Can you work these out from the model? Positions are in its coordinate system, mm. A direction names the side the tool comes from. Coordinates: 2 decimals unless noted, no trailing zeros. Order: outer loops, then holes, each group sorted by start corner. A loop starts at its lowest first (then second) coordinate and runs counter-clockwise, first axis right, second up. Notation, with made-up numbers: (29.25, -21.5) -> (83.25, -21.5) arc R24 cw to (83.25, -2.5) -> close; hole circle Ø1 at (63.5, -13.5). An arc over 180 degrees is marked (long way). Use a Markdown table: item, result. Add a question column.
1. Suppose I cut it at A-A, the plane z = 4. List the corners of the cut face in (x, y) for me.
2. We'd pull the mould along X, two halves only. Please class faces 1 (the flat face through (-0.4, 19, 44.4)), 2 (the flat face through (2, 13, 19.05)), 3 (the flat face through (-51.863, 13, 31)): pulls with the +X half, pulls with the -X half, needs draft (parallel to the pull), parting line crosses it, or undercut.
3. For pin 1 Ø1 at (y, z) = (-6, 31) entering from +X; pin 2 Ø21 at (y, z) = (30, 12.5) entering from +X; pin 3 Ø7.5 at (x, y) = (61, 32) entering from +Z; pin 4 Ø12 at (x, z) = (-9.5, 12.5) entering from -Y (1 decimal), each with a flat end and sliding along its axis, tell me the tip position at first contact or that it passes through.
4. Suppose I cut it at B-B, the plane x = 58. List the corners of the cut face in (y, z) for me, then the cut area to 3 significant figures.
5. For faces 4 (the flat face through (59, 41, 12.7)), 5 (the flat face through (62.62, -12.88, 6.26)), 6 (the flat face through (-34.61, 13, 9)), which set-ups out of +Z, -Z, +X, -X, +Y, -Y let a thin tool reach every point of the face, with its end or its side?
6. Suppose I cut it at D-D, the plane x = -38.5. List the corners of the cut face in (y, z) for me.
7. Suppose I cut it at C-C, the plane y = 1.5. List the corners of the cut face in (x, z) for me, then the cut area to 3 significant figures.
8. If I drill on line 1 along X through (y, z) = (2, 14.5); line 2 along X through (y, z) = (-21.5, 35); line 3 along Z through (x, y) = (-59, -8), over which ranges is the centre line in solid material (lowest first)? Write a range as from..to.
```python
from build123d import *

# Parameters (mm, degrees)
F0_W     = 20.847595
F0_H     = 76.2
F1_DEPTH = 12.7
F2_DEPTH = 50.8
F3_DEPTH = 12.7
F4_DEPTH = 12.7
F6_DEPTH = 122.448595
F7_W     = 71.647595
F7_H     = 19.05
F8_DEPTH = 101.6


with BuildPart() as f1:
    # F0 (on Top) → F1 (new body)
    with BuildSketch(Plane.XY):
        with Locations((-62.286463, 12.7)):
            Rectangle(F0_W, F0_H)
    extrude(amount=F1_DEPTH)

    # F0 (on Top) → F2 (join)
    with BuildSketch(Plane.XY):
        Polygon((49.737334, 50.8), (-51.862666, 50.8), (-51.862666, -25.4), (49.737334, -25.4), (49.737334, 0), (49.737334, 25.4), align=None)
    extrude(amount=F2_DEPTH)

    # F0 (on Top) → F3 (join)
    with BuildSketch(Plane.XY):
        Polygon((75.137334, 50.8), (49.737334, 50.8), (49.737334, 25.4), align=None)
    extrude(amount=F3_DEPTH)

    # F0 (on Top) → F4 (join)
    with BuildSketch(Plane.XY):
        Polygon((49.737334, 0), (49.737334, -25.4), (75.137334, -25.4), align=None)
    extrude(amount=F4_DEPTH)

    # F5 (on face) → F6 (cut, through all)
    with BuildSketch(Plane.YZ.offset(49.737334)):
        Polygon((25.4, 50.8), (0, 50.8), (12.7, 38.1), align=None)
    extrude(amount=-F6_DEPTH, mode=Mode.SUBTRACT)

    # F7 (on face) → F8 (cut)
    with BuildSketch(Plane(origin=(0, 50.8, 0), x_dir=(-1, 0, 0), z_dir=(0, 1, 0))):
        with Locations((-1.213537, 9.525)):
            Rectangle(F7_W, F7_H)
    extrude(amount=-F8_DEPTH, mode=Mode.SUBTRACT)


solid = f1.part
```
Worked out:
| question | item | result |
|---|---|---|
| 1 | outline | (-72.71, -25.4) -> (-34.61, -25.4) -> (-34.61, 50.8) -> (-72.71, 50.8) -> close; (37.04, -25.4) -> (75.14, -25.4) -> (49.74, 0) -> (49.74, 25.4) -> (75.14, 50.8) -> (37.04, 50.8) -> close |
| 2 | face 1 | needs draft |
| 2 | face 2 | undercut |
| 2 | face 3 | pulls with the -X half |
| 3 | pin 1 | stops at x = 49.74 |
| 3 | pin 2 | stops at x = 64.84 |
| 3 | pin 3 | stops at z = 12.7 |
| 3 | pin 4 | passes through |
| 4 | outline | (-25.4, 0) -> (-8.26, 0) -> (-8.26, 12.7) -> (-25.4, 12.7) -> close; (33.66, 0) -> (50.8, 0) -> (50.8, 12.7) -> (33.66, 12.7) -> close |
| 4 | area | 435 mm² |
| 5 | face 4 | +Z, +X, +Y, -Y |
| 5 | face 5 | +Z, -Z, +X |
| 5 | face 6 | -Z, +Y, -Y |
| 6 | outline | (-25.4, 0) -> (50.8, 0) -> (50.8, 50.8) -> (25.4, 50.8) -> (12.7, 38.1) -> (0, 50.8) -> (-25.4, 50.8) -> close |
| 7 | outline | (-72.71, 0) -> (-34.61, 0) -> (-34.61, 19.05) -> (37.04, 19.05) -> (37.04, 0) -> (49.74, 0) -> (49.74, 49.3) -> (-51.86, 49.3) -> (-51.86, 12.7) -> (-72.71, 12.7) -> close |
| 7 | area | 3,910 mm² |
| 8 | line 1 | x = -51.86..-34.61, 37.04..49.74 |
| 8 | line 2 | x = -51.86..49.74 |
| 8 | line 3 | z = 0..12.7 |
